Verification items for the finished model (mm, model axes). Round coordinates to 2 decimals unless told otherwise and drop trailing zeros. Write each loop counter-clockwise with the first axis right and the second up, starting at its lowest first coordinate (ties: lowest second). Pieces come first, ordered by that corner, then holes. Notation, with made-up numbers: (38, 9) - (77, 9) arc R24 cw to (77, 47) - close; hole circle Ø4 at (37.25, 34). An arc over 180 degrees is marked (long way). Answer as a JSON object with one key per item and string values. Group by question number.
1) Section check C-C (z = 0). Enter the section's corners in (x, y).
2) Section check B-B (x = 0). Enter the section's corners in (y, z).
3) Mould release check, pull along Z, two halves, no side actions. Record for faces 1 (the cylindrical face through (28, 2, 29)), 2 (the flat face through (0, 1, -30)), 3 (the cylindrical face through (4.01, 1.48, 18.06)): +Z half, -Z half, draft (parallel to the pull), parting line (faces both ways), or undercut.
4) Section check A-A (y = 0.9). Enter the section's corners in (x, z).
5) Thickness scan on line 1 (Z direction, x = 0, y = 1.95); line 2 (Z direction, x = -9, y = 2.35); line 3 (X direction, y = 2.5, z = 5.5). Record the ranges inside material, lowest first.
Autodesk Inventor part; units mm, degrees
ref_plane "YZ Plane" through (0, 0, 0) normal (1, 0, 0) x (0, 1, 0)
ref_plane "XZ Plane" through (0, 0, 0) normal (0, 1, 0) x (-1, 0, 0)
ref_plane "XY Plane" through (0, 0, 0) normal (0, 0, 1) x (1, 0, 0)
sketch "Sketch1" plane through (0, 0, 0) normal (0, 1, 0) x (-1, 0, 0)
  circle A0 centre (0, 0) radius 18.5
  line L0 (30, 30) -> (-30, 30)
  line L1 (-30, 30) -> (-30, -30)
  line L2 (-30, -30) -> (30, -30)
  line L3 (30, -30) -> (30, 30)
  line L4 (30, 30) -> (-30, -30) construction
  line L5 (-30, 30) -> (30, -30) construction
  dimension "d0" = 37
  dimension "d1" = 60
  dimension "d2" = 60
extrude "Extrusion1" add sketch "Sketch1" along normal blind 3
fillet "Fillet1" radius 5 4 edges at (30, 1.5, 30) (30, 1.5, -30) (-30, 1.5, -30) (-30, 1.5, 30)
properties part number "rimsa"
Returned:
{
 "1": {"outline": "(-30, 0) - (-18.5, 0) - (-18.5, 3) - (-30, 3) - close; (18.5, 0) - (30, 0) - (30, 3) - (18.5, 3) - close"},
 "2": {"outline": "(0, -30) - (3, -30) - (3, -18.5) - (0, -18.5) - close; (0, 18.5) - (3, 18.5) - (3, 30) - (0, 30) - close"},
 "3": {"face 1": "+Z half", "face 2": "-Z half", "face 3": "undercut"},
 "4": {"outline": "(-30, -25) arc R5 ccw to (-25, -30) - (25, -30) arc R5 ccw to (30, -25) - (30, 25) arc R5 ccw to (25, 30) - (-25, 30) arc R5 ccw to (-30, 25) - close; hole circle Ø37 at (0, 0)"},
 "5": {"line 1": "-30 to -18.5, 18.5 to 30", "line 2": "-30 to -16.16, 16.16 to 30", "line 3": "-30 to -17.66, 17.66 to 30"}
}
